Part model, mm, in its own coordinate system. A direction names the side the tool comes from. Round coordinates to 2 decimals unless told otherwise and drop trailing zeros. Write each loop counter-clockwise with the first axis right and the second up, starting at its lowest first coordinate (ties: lowest second). Pieces come first, ordered by that corner, then holes.
1) Which spindle directions (+Z, -Z, +X, -X, +Y, -Y) get a long thin tool onto all of the face, cutting with end or side? Do faces 1 (the flat face through (0, 10, -1.5)), 2 (the flat face through (-2, 27, 2)), 3 (the flat face through (2, 27, 2)), 4 (the flat face through (-4, 21, 2)). Say none if no direction does.
2) Pull direction Y, two halves, no side cores. Call faces 5 (the cylindrical face through (-0.69, 17.9, 2.99)), 6 (the flat face through (0, 17, 2)), 7 (the cylindrical face through (0.69, -3.1, -0.02)): +Y half, -Y half, draft (parallel to the pull), parting line (faces both ways), or undercut.
3) Flat gauge pins, fed straight in: pin 1 (1.5 mm diameter, centred on x = 4.5, y = 18.5, fed in from -Z); pin 2 (0.8 mm diameter, centred on x = -1, z = 2, fed in from -Y); pin 3 (2 mm diameter, centred on y = 26.5, z = -0.5, fed in from +X). Where does each tip first touch, or does it go through?
4) Saw through at D-D on x = -2.75. Write the cut outline in (y, z).
5) Drill centre lines: L1, parallel to Y at x = 0, z = 0.8 (3 decimals); L2, parallel to Y at x = 0, z = -0.4 (3 decimals); L3, parallel to Z at x = 1.25, y = 27.25. Where is each one in solid material? Low to high.
6) Saw through at A-A on x = 0. Count the separate pieces of the cut face and the enclosed holes in it, and give its area (3 significant figures).
7) Saw through at B-B on y = 27.25. Write the cut outline in (x, z), and give its area (3 significant figures).
```python
from build123d import *

# Parameters (mm, degrees)
F1_DEPTH = 1.5
F2_W     = 8
F2_H     = 8
F3_DEPTH = 1
F4_R     = 3.175
F5_DEPTH = 1
F7_DEPTH = 2
F9_D     = 3.175
F11_D    = 6.35


with BuildPart() as f1:
    # F0 (on Top) → F1 (new body, symmetric)
    with BuildSketch(Plane.XY):
        with BuildLine():
            Line((-6.5, 25), (-6.5, 0))
            ThreePointArc((-6.5, 0), (0, -6.5), (6.5, 0))
            Line((6.5, 0), (6.5, 25))
            Line((6.5, 25), (-6.5, 25))
        make_face()
    extrude(amount=F1_DEPTH, both=True)

    # F2 (on face) → F3 (join)
    with BuildSketch(Plane.XY.offset(1.5)):
        with Locations((0, 21)):
            Rectangle(F2_W, F2_H)
    extrude(amount=F3_DEPTH)

    # F4 (on face) → F5 (join)
    with BuildSketch(Plane.XY.offset(2.5)):
        with Locations((0, 21)):
            Circle(F4_R)
    extrude(amount=F5_DEPTH)

    # F6 (on Right) → F7 (join, symmetric)
    with BuildSketch(Plane.YZ):
        with BuildLine():
            Line((25.572949, 1.5), (25, 1.5))
            Line((25, 1.5), (25, -1.5))
            Line((25, -1.5), (25.572949, -1.5))
            ThreePointArc((25.572949, -1.5), (29.5, 0), (25.572949, 1.5))
        make_face()
    extrude(amount=F7_DEPTH, both=True)

    # F9 (through all)
    with Locations(Plane.YZ.offset(2)):
        with Locations((27.25, 0)):
            Hole(F9_D / 2)

    # F11 (through all)
    with Locations(Plane.XY.offset(1.5)):
        with Locations((0, 0)):
            Hole(F11_D / 2)


solid = f1.part
```
Completed:
1. face 1: -Z, +X, -X, -Y
1. face 2: +Z, -Z, -X, +Y
1. face 3: +Z, -Z, +X, +Y
1. face 4: +Z, -X, +Y, -Y
2. face 5: parting line
2. face 6: -Y half
2. face 7: undercut
3. pin 1: stops at z = -1.5
3. pin 2: stops at y = 17
3. pin 3: stops at x = 2
4. outline: (-5.89, -1.5) - (-1.59, -1.5) - (-1.59, 1.5) - (-5.89, 1.5) - close; (1.59, -1.5) - (25, -1.5) - (25, 2.5) - (22.59, 2.5) - (22.59, 3.5) - (19.41, 3.5) - (19.41, 2.5) - (17, 2.5) - (17, 1.5) - (1.59, 1.5) - close
5. L1: y = -6.5 to -3.175, 3.175 to 25.879, 28.621 to 29.353
5. L2: y = -6.5 to -3.175, 3.175 to 25.714, 28.786 to 29.464
5. L3: z = -2.25 to -1.59, 1.59 to 2.25
6. separate pieces: 2
6. enclosed holes: 1
6. area: 98.3 mm2
7. outline: (-2, -2.25) - (2, -2.25) - (2, -1.59) - (-2, -1.59) - close; (-2, 1.59) - (2, 1.59) - (2, 2.25) - (-2, 2.25) - close
7. area: 5.30 mm2
